The listing builds one solid part. Answer for the finished solid, in the listing's coordinates (mm). A direction names the side the tool comes from. Give positions to 0.01 mm unless a question says otherwise; leave off trailing zeros. Order: outer loops, then holes, each group sorted by start corner. A loop starts at its lowest first (then second) coordinate and runs counter-clockwise, first axis right, second up. Notation, with made-up numbers: (-30.5, 19.25) - (-6.5, 19.25) arc R20 ccw to (-6.5, 25.25) - close; hole circle Ø1 at (-38.75, 64). An arc over 180 degrees is marked (long way). Use a Markdown table: item, result. Add a question column.
1) The mould has two halves that part along Y. Classify faces 4 (the face through (2, 2, 45)), 5 (the face through (-4, 8.2, 1)), 6 (the face through (9.575, 9.551, 0.63)): released by +Y, released by -Y, zero draft, split by the parting line, or undercut.
2) Straight lines are drawn through the part: line 1 (Y direction, x = -5, z = 5); line 2 (Y direction, x = 0, z = -19.5); line 3 (X direction, y = 3.5, z = 0). For each, find the intervals that lie inside material, in ascending order.
3) For faces 1 (the face through (-3.9, 0, 1)), 2 (the face through (0, -3.9, 1)), 3 (the face through (-8.2, 4, 1)), determine the directions among +Z, -Z, +X, -X, +Y, -Y from which every point of the face is accessible in a straight line to the end or side of a thin tool.
4) Find section A-A, the plane y = 0. Determine the outline of the cut face in (x, z).
5) Flat-ended cylindrical pins translate along their axes: pin 1 (4 mm diameter, centred on x = 0, y = 0, fed in from +Z); pin 2 (2 mm diameter, centred on x = 0.5, z = 20, fed in from -Y). Find the tip coordinate at first contact, or state that the pin passes through.
from build123d import *

# Parameters (mm, degrees)
SKETCH_1_R      = 2.5
EXTRUDE_1_DEPTH = 45


with BuildPart() as part:
    # 草图1 → 凸台-拉伸1 (new, symmetric)
    with BuildSketch(Plane.XY):
        with BuildLine():
            Line((-8.502261885, -10.002261885), (-3.85, -10.002261885))
            ThreePointArc((-3.85, -10.002261885), (-3.673223305, -9.929038581), (-3.6, -9.752261885))
            Line((-3.6, -9.752261885), (-3.6, -9.502261885))
            Line((-3.6, -9.502261885), (-3.35, -9.502261885))
            ThreePointArc((-3.35, -9.502261885), (-3.173223305, -9.429038581), (-3.1, -9.252261885))
            Line((-3.1, -9.252261885), (-3.1, -8.45))
            ThreePointArc((-3.1, -8.45), (-3.173223305, -8.273223305), (-3.35, -8.2))
            Line((-3.35, -8.2), (-5.25, -8.2))
            ThreePointArc((-5.25, -8.2), (-5.426776695, -8.126776695), (-5.5, -7.95))
            Line((-5.5, -7.95), (-5.5, -6.664213562))
            ThreePointArc((-5.5, -6.664213562), (-5.480969883, -6.568542704), (-5.426776695, -6.487436867))
            Line((-5.426776695, -6.487436867), (-3.278679656, -4.339339828))
            ThreePointArc((-3.278679656, -4.339339828), (-2.792044633, -4.014180701), (-2.218019485, -3.9))
            Line((-2.218019485, -3.9), (2.218019485, -3.9))
            ThreePointArc((2.218019485, -3.9), (2.792044633, -4.014180701), (3.278679656, -4.339339828))
            Line((3.278679656, -4.339339828), (5.426776695, -6.487436867))
            ThreePointArc((5.426776695, -6.487436867), (5.480969883, -6.568542704), (5.5, -6.664213562))
            Line((5.5, -6.664213562), (5.5, -7.95))
            ThreePointArc((5.5, -7.95), (5.426776695, -8.126776695), (5.25, -8.2))
            Line((5.25, -8.2), (3.35, -8.2))
            ThreePointArc((3.35, -8.2), (3.173223305, -8.273223305), (3.1, -8.45))
            Line((3.1, -8.45), (3.1, -9.252261885))
            ThreePointArc((3.1, -9.252261885), (3.173223305, -9.429038581), (3.35, -9.502261885))
            Line((3.35, -9.502261885), (3.6, -9.502261885))
            Line((3.6, -9.502261885), (3.6, -9.752261885))
            ThreePointArc((3.6, -9.752261885), (3.673223305, -9.929038581), (3.85, -10.002261885))
            Line((3.85, -10.002261885), (8.502261885, -10.002261885))
            ThreePointArc((8.502261885, -10.002261885), (9.562922057, -9.562922057), (10.002261885, -8.502261885))
            Line((10.002261885, -8.502261885), (10.002261885, -3.85))
            ThreePointArc((10.002261885, -3.85), (9.929038581, -3.673223305), (9.752261885, -3.6))
            Line((9.752261885, -3.6), (9.502261885, -3.6))
            Line((9.502261885, -3.6), (9.502261885, -3.35))
            ThreePointArc((9.502261885, -3.35), (9.429038581, -3.173223305), (9.252261885, -3.1))
            Line((9.252261885, -3.1), (8.45, -3.1))
            ThreePointArc((8.45, -3.1), (8.273223305, -3.173223305), (8.2, -3.35))
            Line((8.2, -3.35), (8.2, -5.25))
            ThreePointArc((8.2, -5.25), (8.126776695, -5.426776695), (7.95, -5.5))
            Line((7.95, -5.5), (6.664213562, -5.5))
            ThreePointArc((6.664213562, -5.5), (6.568542704, -5.480969883), (6.487436867, -5.426776695))
            Line((6.487436867, -5.426776695), (4.339339828, -3.278679656))
            ThreePointArc((4.339339828, -3.278679656), (4.014180701, -2.792044633), (3.9, -2.218019485))
            Line((3.9, -2.218019485), (3.9, 2.218019485))
            ThreePointArc((3.9, 2.218019485), (4.014180701, 2.792044633), (4.339339828, 3.278679656))
            Line((4.339339828, 3.278679656), (6.487436867, 5.426776695))
            ThreePointArc((6.487436867, 5.426776695), (6.568542704, 5.480969883), (6.664213562, 5.5))
            Line((6.664213562, 5.5), (7.95, 5.5))
            ThreePointArc((7.95, 5.5), (8.126776695, 5.426776695), (8.2, 5.25))
            Line((8.2, 5.25), (8.2, 3.35))
            ThreePointArc((8.2, 3.35), (8.273223305, 3.173223305), (8.45, 3.1))
            Line((8.45, 3.1), (9.252261885, 3.1))
            ThreePointArc((9.252261885, 3.1), (9.429038581, 3.173223305), (9.502261885, 3.35))
            Line((9.502261885, 3.35), (9.502261885, 3.6))
            Line((9.502261885, 3.6), (9.752261885, 3.6))
            ThreePointArc((9.752261885, 3.6), (9.929038581, 3.673223305), (10.002261885, 3.85))
            Line((10.002261885, 3.85), (10.002261885, 8.502261885))
            ThreePointArc((10.002261885, 8.502261885), (9.562922057, 9.562922057), (8.502261885, 10.002261885))
            Line((8.502261885, 10.002261885), (3.85, 10.002261885))
            ThreePointArc((3.85, 10.002261885), (3.673223305, 9.929038581), (3.6, 9.752261885))
            Line((3.6, 9.752261885), (3.6, 9.502261885))
            Line((3.6, 9.502261885), (3.35, 9.502261885))
            ThreePointArc((3.35, 9.502261885), (3.173223305, 9.429038581), (3.1, 9.252261885))
            Line((3.1, 9.252261885), (3.1, 8.45))
            ThreePointArc((3.1, 8.45), (3.173223305, 8.273223305), (3.35, 8.2))
            Line((3.35, 8.2), (5.25, 8.2))
            ThreePointArc((5.25, 8.2), (5.426776695, 8.126776695), (5.5, 7.95))
            Line((5.5, 7.95), (5.5, 6.664213562))
            ThreePointArc((5.5, 6.664213562), (5.480969883, 6.568542704), (5.426776695, 6.487436867))
            Line((5.426776695, 6.487436867), (3.278679656, 4.339339828))
            ThreePointArc((3.278679656, 4.339339828), (2.792044633, 4.014180701), (2.218019485, 3.9))
            Line((2.218019485, 3.9), (-2.218019485, 3.9))
            ThreePointArc((-2.218019485, 3.9), (-2.792044633, 4.014180701), (-3.278679656, 4.339339828))
            Line((-3.278679656, 4.339339828), (-5.426776695, 6.487436867))
            ThreePointArc((-5.426776695, 6.487436867), (-5.480969883, 6.568542704), (-5.5, 6.664213562))
            Line((-5.5, 6.664213562), (-5.5, 7.95))
            ThreePointArc((-5.5, 7.95), (-5.426776695, 8.126776695), (-5.25, 8.2))
            Line((-5.25, 8.2), (-3.35, 8.2))
            ThreePointArc((-3.35, 8.2), (-3.173223305, 8.273223305), (-3.1, 8.45))
            Line((-3.1, 8.45), (-3.1, 9.252261885))
            ThreePointArc((-3.1, 9.252261885), (-3.173223305, 9.429038581), (-3.35, 9.502261885))
            Line((-3.35, 9.502261885), (-3.6, 9.502261885))
            Line((-3.6, 9.502261885), (-3.6, 9.752261885))
            ThreePointArc((-3.6, 9.752261885), (-3.673223305, 9.929038581), (-3.85, 10.002261885))
            Line((-3.85, 10.002261885), (-8.502261885, 10.002261885))
            ThreePointArc((-8.502261885, 10.002261885), (-9.562922057, 9.562922057), (-10.002261885, 8.502261885))
            Line((-10.002261885, 8.502261885), (-10.002261885, 3.85))
            ThreePointArc((-10.002261885, 3.85), (-9.929038581, 3.673223305), (-9.752261885, 3.6))
            Line((-9.752261885, 3.6), (-9.502261885, 3.6))
            Line((-9.502261885, 3.6), (-9.502261885, 3.35))
            ThreePointArc((-9.502261885, 3.35), (-9.429038581, 3.173223305), (-9.252261885, 3.1))
            Line((-9.252261885, 3.1), (-8.45, 3.1))
            ThreePointArc((-8.45, 3.1), (-8.273223305, 3.173223305), (-8.2, 3.35))
            Line((-8.2, 3.35), (-8.2, 5.25))
            ThreePointArc((-8.2, 5.25), (-8.126776695, 5.426776695), (-7.95, 5.5))
            Line((-7.95, 5.5), (-6.664213562, 5.5))
            ThreePointArc((-6.664213562, 5.5), (-6.568542704, 5.480969883), (-6.487436867, 5.426776695))
            Line((-6.487436867, 5.426776695), (-4.339339828, 3.278679656))
            ThreePointArc((-4.339339828, 3.278679656), (-4.014180701, 2.792044633), (-3.9, 2.218019485))
            Line((-3.9, 2.218019485), (-3.9, -2.218019485))
            ThreePointArc((-3.9, -2.218019485), (-4.014180701, -2.792044633), (-4.339339828, -3.278679656))
            Line((-4.339339828, -3.278679656), (-6.487436867, -5.426776695))
            ThreePointArc((-6.487436867, -5.426776695), (-6.568542704, -5.480969883), (-6.664213562, -5.5))
            Line((-6.664213562, -5.5), (-7.95, -5.5))
            ThreePointArc((-7.95, -5.5), (-8.126776695, -5.426776695), (-8.2, -5.25))
            Line((-8.2, -5.25), (-8.2, -3.35))
            ThreePointArc((-8.2, -3.35), (-8.273223305, -3.173223305), (-8.45, -3.1))
            Line((-8.45, -3.1), (-9.252261885, -3.1))
            ThreePointArc((-9.252261885, -3.1), (-9.429038581, -3.173223305), (-9.502261885, -3.35))
            Line((-9.502261885, -3.35), (-9.502261885, -3.6))
            Line((-9.502261885, -3.6), (-9.752261885, -3.6))
            ThreePointArc((-9.752261885, -3.6), (-9.929038581, -3.673223305), (-10.002261885, -3.85))
            Line((-10.002261885, -3.85), (-10.002261885, -8.502261885))
            ThreePointArc((-10.002261885, -8.502261885), (-9.562922057, -9.562922057), (-8.502261885, -10.002261885))
        make_face()
        with Locations(Location((0, 0, 0), (0, 0, 180))):
            Circle(SKETCH_1_R, mode=Mode.SUBTRACT)
    extrude(amount=EXTRUDE_1_DEPTH, both=True)


solid = part.part
The answers:
| question | item | result |
|---|---|---|
| 1 | face 4 | zero draft |
| 1 | face 5 | undercut |
| 1 | face 6 | released by +Y |
| 2 | line 1 | -10 to -8.2, -6.06 to -3.94, 3.94 to 6.06, 8.2 to 10 |
| 2 | line 2 | -3.9 to -2.5, 2.5 to 3.9 |
| 2 | line 3 | -9.5 to -8.2, -4.56 to 4.56, 8.2 to 9.5 |
| 3 | face 1 | +Z, -Z, -X |
| 3 | face 2 | +Z, -Z, -Y |
| 3 | face 3 | +Z, -Z |
| 4 | outline | (-3.9, -45) - (-2.5, -45) - (-2.5, 45) - (-3.9, 45) - close; (2.5, -45) - (3.9, -45) - (3.9, 45) - (2.5, 45) - close |
| 5 | pin 1 | through |
| 5 | pin 2 | y = -3.9 |
